For this review, use the dimensioned drawing (mm, ordinates from the lowest corner) and the shaded views. A direction names the side the tool comes from. Give positions to 0.01 mm unless a question says otherwise; leave off trailing zeros. Loops run counter-clockwise (first coordinate to the right, second up) from the corner with the lowest first, then second, coordinate; pieces in that order, holes last. Notation, with made-up numbers: (87.25, 67.5) -> (93.25, 67.5) arc R21 ccw to (93.25, 84.5) -> close; hole circle Ø1 at (75, -13.75). An arc over 180 degrees is marked (long way). Use a Markdown table: item, result. Add a question column.
1. Add section C-C (x = 64.5). State the section outline as (y, z) points.
2. Add section B-B (z = 23.5). State the section outline as (x, y) points (3 decimals).
3. For the marked faces 5 and 6, list the 3-axis set-ups (+Z, -Z, +X, -X, +Y, -Y) from which the entire face can be reached by the end or side of a thin tool; tool diameter is ignored.
4. Draft analysis for pull direction X (two halves, no side actions). For the marked faces 1, 2, 3 and 4, state which applies: pulls with the +X half, pulls with the -X half, needs draft (parallel to the pull), parting line crosses it, or undercut.
5. Add section A-A (y = 44.5). State the section outline as (x, z) points, and give its area (3 significant figures).
6. To check wall thickness, follow line 1 (X direction, y = 39, z = 8.75); line 2 (Y direction, x = 40, z = 20); line 3 (Y direction, x = 75, z = 2). State the ranges of each line that lie inside material, in increasing order.
7. Add section D-D (y = 27). State the section outline as (x, z) points, and give its area (3 significant figures).
8. For pin 1 Ø4 at (x, z) = (44.5, 3) entering from +Y; pin 2 Ø12 at (x, y) = (30, 7.5) entering from -Z, all flat-tipped, find the tip position at first contact; note any pin that passes through.
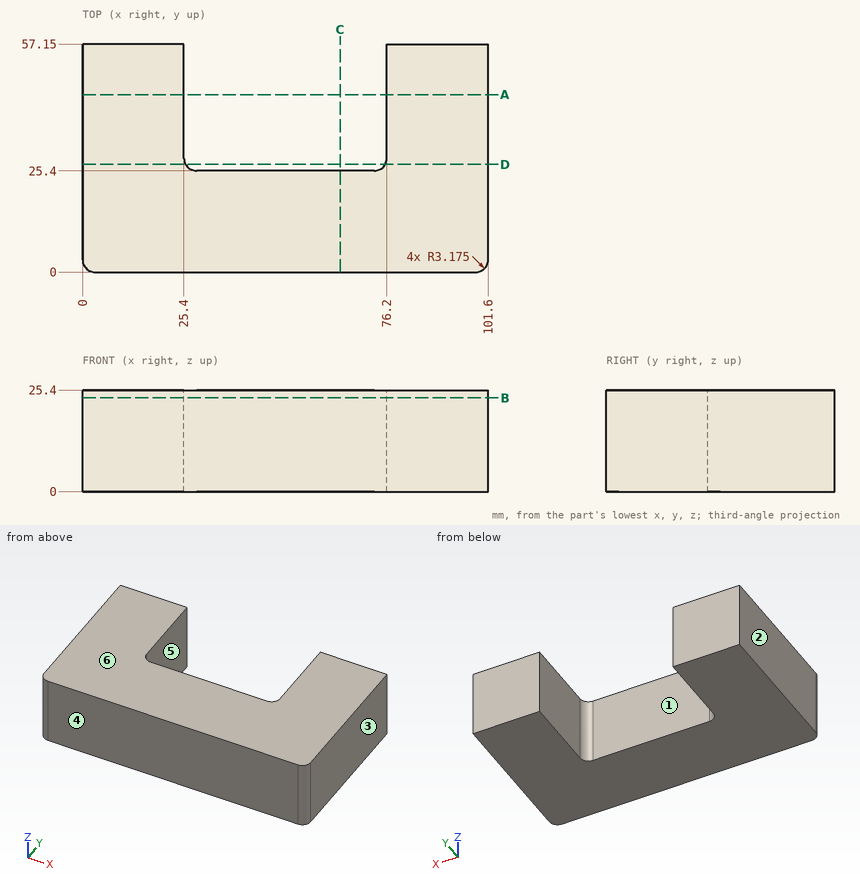
Taken from the geometry:
| question | item | result |
|---|---|---|
| 1 | outline | (0, 0) -> (25.4, 0) -> (25.4, 25.4) -> (0, 25.4) -> close |
| 2 | outline | (0, 3.175) arc R3.175 ccw to (3.175, 0) -> (98.425, 0) arc R3.175 ccw to (101.6, 3.175) -> (101.6, 57.15) -> (76.2, 57.15) -> (76.2, 28.575) arc R3.175 cw to (73.025, 25.4) -> (28.575, 25.4) arc R3.175 cw to (25.4, 28.575) -> (25.4, 57.15) -> (0, 57.15) -> close |
| 3 | face 5 | +Z, -Z, +Y |
| 3 | face 6 | +Z, +X, -X, +Y, -Y |
| 4 | face 1 | undercut |
| 4 | face 2 | pulls with the -X half |
| 4 | face 3 | pulls with the +X half |
| 4 | face 4 | needs draft |
| 5 | outline | (0, 0) -> (25.4, 0) -> (25.4, 25.4) -> (0, 25.4) -> close; (76.2, 0) -> (101.6, 0) -> (101.6, 25.4) -> (76.2, 25.4) -> close |
| 5 | area | 1,290 mm^2 |
| 6 | line 1 | x = 0 to 25.4, 76.2 to 101.6 |
| 6 | line 2 | y = 0 to 25.4 |
| 6 | line 3 | y = 0 to 26.09 |
| 7 | outline | (0, 0) -> (25.82, 0) -> (25.82, 25.4) -> (0, 25.4) -> close; (75.78, 0) -> (101.6, 0) -> (101.6, 25.4) -> (75.78, 25.4) -> close |
| 7 | area | 1,310 mm^2 |
| 8 | pin 1 | stops at y = 25.4 |
| 8 | pin 2 | stops at z = 0 |
